from build123d import *

# Parameters (mm, degrees)
SKETCH_1_W                   = 75
SKETCH_1_H                   = 92
EXTRUDE_460_DEPTH            = 5
HOLE_WIZARD_M3_D             = 2.5
HOLE_WIZARD_M3_2_D           = 3.4
HOLE_WIZARD_M3_2_CSINK_D     = 6.3
HOLE_WIZARD_M3_2_CSINK_ANGLE = 90
SKETCH_6_W                   = 7
SKETCH_6_H                   = 80
CUT_EXTRUDE_1_DEPTH          = 1


with BuildPart() as part:
    # Эскиз1 → Extrude 460 (new body)
    with BuildSketch(Plane.XY):
        Rectangle(SKETCH_1_W, SKETCH_1_H)
    extrude(amount=-EXTRUDE_460_DEPTH)

    # Hole Wizard M3 (through all)
    with Locations(Plane(origin=(0, 46, 0), x_dir=(1, 0, 0), z_dir=(0, 1, 0))):
        with Locations((30, 2.5), (-30, 2.5), (0, 2.5)):
            Hole(HOLE_WIZARD_M3_D / 2)

    # Hole Wizard M3 2 (through all)
    with Locations(Plane(origin=(45, 0, 0), x_dir=(-1, 0, 0), z_dir=(0, 0, 1))):
        with Locations((10.5, 0), (10.5, -33.5), (10.5, 33.5), (79.5, -33.5), (79.5, 0), (79.5, 33.5)):
            CounterSinkHole(HOLE_WIZARD_M3_2_D / 2, HOLE_WIZARD_M3_2_CSINK_D / 2, counter_sink_angle=HOLE_WIZARD_M3_2_CSINK_ANGLE)

    # Эскиз6 → Вырез-Вытянуть1 (cut)
    with BuildSketch(Plane.XY):
        Rectangle(SKETCH_6_W, SKETCH_6_H)
    extrude(amount=-CUT_EXTRUDE_1_DEPTH, mode=Mode.SUBTRACT)


solid = part.part
CAD build for the part. Positions are in the model's coordinates, mm. Coordinates: 2 decimals unless noted, no trailing zeros. Loops run counter-clockwise (first coordinate to the right, second up) from the corner with the lowest first, then second, coordinate; pieces in that order, holes last. Notation, with made-up numbers: (54, 6.25) -> (100, 6.25) arc R24 ccw to (100, 41.25) -> close; hole circle Ø11 at (-27.5, 80.25). An arc over 180 degrees is marked (long way). One line per item, written item: value.
1. Slice it at D-D on x = 0. Write the cut outline in (y, z).
Answers:
outline: (-46, -5) -> (46, -5) -> (46, -3.75) -> (-46, -3.75) -> close; (-46, -1.25) -> (46, -1.25) -> (46, 0) -> (40, 0) -> (40, -1) -> (-40, -1) -> (-40, 0) -> (-46, 0) -> close
2. Slice it at C-C on y = 38.5. Write the cut outline in (x, z).
Answers:
outline: (-37.5, -5) -> (37.5, -5) -> (37.5, 0) -> (3.5, 0) -> (3.5, -1) -> (-3.5, -1) -> (-3.5, 0) -> (-37.5, 0) -> close; hole circle Ø2.5 at (-30, -2.5); hole circle Ø2.5 at (0, -2.5); hole circle Ø2.5 at (30, -2.5)
3. Slice it at B-B on x = 30. Write the cut outline in (y, z), and give its area (3 significant figures).
Answers:
outline: (-46, -5) -> (46, -5) -> (46, -3.75) -> (-46, -3.75) -> close; (-46, -1.25) -> (46, -1.25) -> (46, 0) -> (-46, 0) -> close
area: 230 mm^2
4. Pull direction Z, two halves, no side cores. Call faces 1 (the face through (0.16, -0.64, -3.74)), 2 (the face through (0, 1, -1)), 3 (the face through (-33.7, 35, -3.2)): pulls with the +Z half, pulls with the -Z half, needs draft (parallel to the pull), parting line crosses it, or undercut.
Answers:
face 1: undercut
face 2: pulls with the +Z half
face 3: needs draft
5. Slice it at A-A on z = -2.5. Give the number of separate pieces and of enclosed holes in the cut face, and give its area (3 significant figures).
Answers:
separate pieces: 4
enclosed holes: 6
area: 6,160 mm^2
6. Drill centre lines: line 1 (Y direction, x = -34.5, z = -2.35); line 2 (X direction, y = -33.5, z = -2.4); line 3 (X direction, y = 4, z = -2.4). Where is each one in solid material? Low to high. Write a range as [from, to].
Answers:
line 1: y = [-46, -35.2], [-31.8, -1.7], [1.7, 31.8], [35.2, 46]
line 2: x = [-37.5, -36.2], [-32.8, -31.25], [-28.75, -1.25], [1.25, 28.75], [31.25, 32.8], [36.2, 37.5]
line 3: x = [-37.5, -31.25], [-28.75, -1.25], [1.25, 28.75], [31.25, 37.5]
7. Flat gauge pins, fed straight in: P1, Ø4.5, axis at x = 34.5, y = 33.5, coming from the +Z side; P2, Ø3.5, axis at x = -1, y = -1.5, coming from the +Z side. Where does each tip first touch, or does it go through?
Answers:
P1: stops at z = -0.9
P2: stops at z = -1
